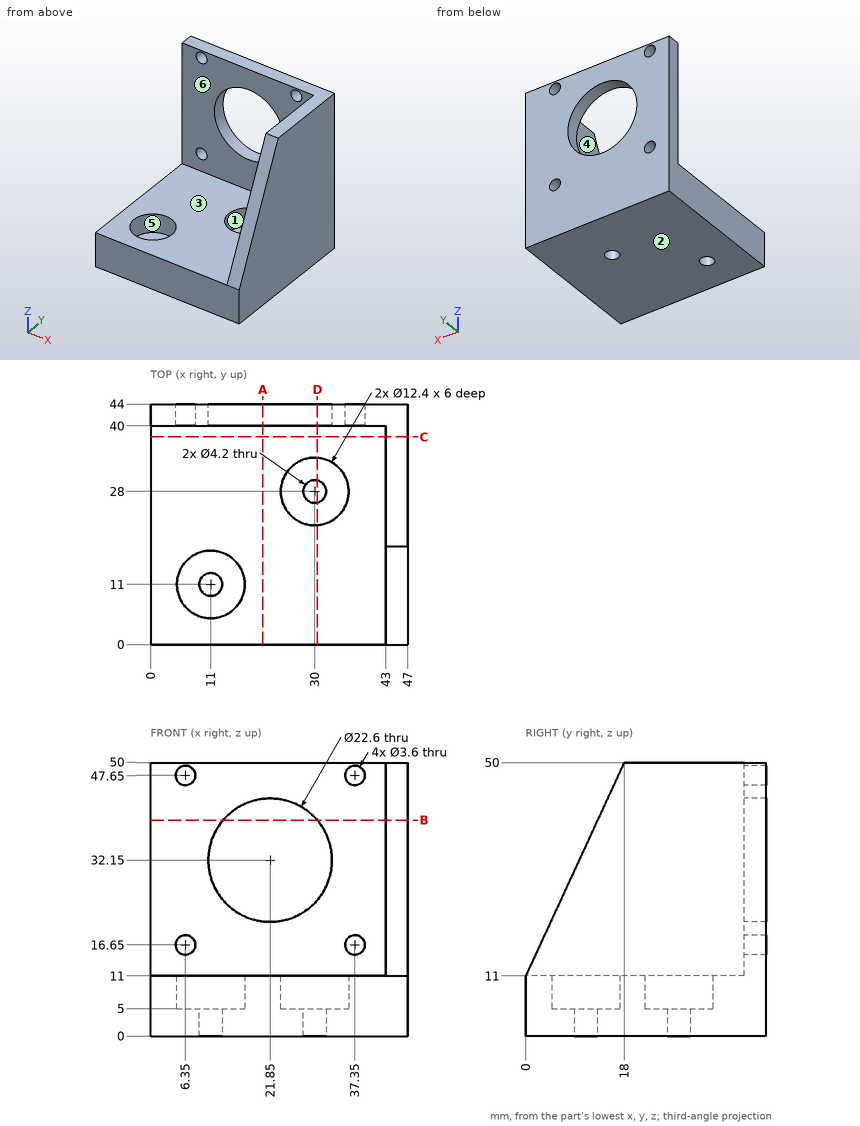
Check sheet for the drawn part. Datum: minimum x, y, z corner. Units: mm. A direction names the side the tool comes from. Round coordinates to 2 decimals unless told otherwise and drop trailing zeros. Order: outer loops, then holes, each group sorted by start corner. A loop starts at its lowest first (then second) coordinate and runs counter-clockwise, first axis right, second up. Notation, with made-up numbers: (81.25, 34.25) -> (86.25, 34.25) arc R11 cw to (86.25, 50.25) -> close; hole circle Ø1 at (-6.5, -30.75). An arc over 180 degrees is marked (long way). Put each result on its own line as item: value. Start each with the question number.
(1) Tool access check on the marked faces 1, 2 and 3. Record the directions out of +Z, -Z, +X, -X, +Y, -Y that give a thin tool (end or side, any length) a straight path to the whole face; none if there is none.
(2) Depth check by flat-ended pin: pin 1 Ø3 at (x, z) = (38, 18.5) entering from -Y; pin 2 Ø5.5 at (x, y) = (11, 11) entering from +Z; pin 3 Ø10 at (x, y) = (27.5, 26.5) entering from +Z; pin 4 Ø4 at (x, z) = (6.35, 16.65) entering from +Y. Enter the tip coordinate at first touch or a pass-through.
(3) Draft check along X on the marked faces 4, 5 and 6. Enter one of: +X half, -X half, draft (parallel to the pull), parting line (faces both ways), or undercut.
(4) Section check D-D (x = 30.5). Enter the section's corners in (y, z).
(5) Material ranges on line 1 along X through (y, z) = (41.4, 47.65); line 2 along Z through (x, y) = (37.35, 41.8); line 3 along Y through (x, z) = (11, 9.45), recorded low to high.
(6) Section check C-C (y = 38). Enter the section's corners in (x, z).
(7) Section check B-B (z = 39.5). Enter the section's corners in (x, y), then the cut area to 3 significant figures.
(8) Section check A-A (x = 20.5). Enter the section's corners in (y, z), then the cut area to 3 significant figures.
Completed:
1. face 1: +Z
1. face 2: -Z, +X, -X, +Y, -Y
1. face 3: +Z, -X, -Y
2. pin 1: stops at y = 40
2. pin 2: stops at z = 5
2. pin 3: stops at z = 11
2. pin 4: stops at y = 44
3. face 4: -X half
3. face 5: undercut
3. face 6: draft
4. outline: (0, 0) -> (25.96, 0) -> (25.96, 5) -> (21.82, 5) -> (21.82, 11) -> (0, 11) -> close; (30.04, 0) -> (44, 0) -> (44, 24.88) -> (40, 24.88) -> (40, 11) -> (34.18, 11) -> (34.18, 5) -> (30.04, 5) -> close; (40, 39.42) -> (44, 39.42) -> (44, 50) -> (40, 50) -> close
5. line 1: x = 0 to 4.55, 8.15 to 35.55, 39.15 to 47
5. line 2: z = 0 to 14.85, 18.45 to 45.85, 49.45 to 50
5. line 3: y = 0 to 4.8, 17.2 to 44
6. outline: (0, 0) -> (47, 0) -> (47, 50) -> (43, 50) -> (43, 11) -> (0, 11) -> close
7. outline: (0, 40) -> (13.27, 40) -> (13.27, 44) -> (0, 44) -> close; (30.43, 40) -> (43, 40) -> (43, 13.15) -> (47, 13.15) -> (47, 44) -> (30.43, 44) -> close
7. area: 227 mm2
8. outline: (0, 0) -> (44, 0) -> (44, 20.93) -> (40, 20.93) -> (40, 11) -> (0, 11) -> close; (40, 43.37) -> (44, 43.37) -> (44, 50) -> (40, 50) -> close
8. area: 550 mm2
